Geometry: final body of the model. Coordinates: model frame, mm. Round coordinates to 2 decimals unless told otherwise and drop trailing zeros. Loops run counter-clockwise (first coordinate to the right, second up) from the corner with the lowest first, then second, coordinate; pieces in that order, holes last. Notation, with made-up numbers: (65.5, -9) -> (85.5, -9) arc R22 cw to (85.5, 12) -> close; hole circle Ø3 at (-29.75, 30.5). An arc over 180 degrees is marked (long way). Answer in a Markdown table with one row per item.
```python
from build123d import *

# Parameters (mm, degrees)
SKETCH1_W           = 67.3
SKETCH1_H           = 135.4
BOSS_EXTRUDE1_DEPTH = 15.1
FILLET1_R           = 5
FILLET2_R           = 3.75
SKETCH2_W           = 12.2
SKETCH2_H           = 4.45
CUT_EXTRUDE1_DEPTH  = 3
SKETCH3_W           = 8.2
SKETCH3_H           = 3.5
SKETCH3_W_2         = 8
SKETCH3_H_2         = 3.3
CUT_EXTRUDE2_DEPTH  = 3
FILLET3_R           = 3.75
SKETCH4_W           = 8
SKETCH4_H           = 3.3
BOSS_EXTRUDE2_DEPTH = 0.5
FILLET4_R           = 0.2
FILLET5_R           = 0.2


with BuildPart() as part:
    # Sketch1 → Boss-Extrude1 (new body)
    with BuildSketch(Plane(origin=(0, 0, 0), x_dir=(1, 0, 0), z_dir=(0, 1, 0))):
        with Locations((33.65, 67.7)):
            Rectangle(SKETCH1_W, SKETCH1_H)
    extrude(amount=BOSS_EXTRUDE1_DEPTH)

    # Fillet1
    fillet1_edges = [part.edges().sort_by_distance(p)[0] for p in [
        (0, 7.55, -135.4),
        (67.3, 7.55, -135.4),
        (67.3, 7.55, 0),
        (0, 7.55, 0),
    ]]
    fillet(fillet1_edges, radius=FILLET1_R)

    # Fillet2
    fillet2_edges = [part.edges().sort_by_distance(p)[0] for p in [
        (0, 15.1, -67.7),
        (33.65, 15.1, -135.4),
        (33.65, 15.1, 0),
        (67.3, 15.1, -67.7),
        (1.464466094, 15.1, -1.464466094),
        (65.835533906, 15.1, -1.464466094),
        (65.835533906, 15.1, -133.935533906),
        (1.464466094, 15.1, -133.935533906),
    ]]
    fillet(fillet2_edges, radius=FILLET2_R)

    # Sketch2 → Cut-Extrude1 (cut)
    with BuildSketch(Plane.XY):
        with Locations((17.1, 8.125)):
            Rectangle(SKETCH2_W, SKETCH2_H)
        with Locations((50.2, 8.125)):
            Rectangle(SKETCH2_W, SKETCH2_H)
        with BuildLine():
            Line((30.2, 7.55), (37.1, 7.55))
            ThreePointArc((37.1, 7.55), (37.807106781, 7.842893219), (38.1, 8.55))
            Line((38.1, 8.55), (38.1, 9.35))
            ThreePointArc((38.1, 9.35), (37.807106781, 10.057106781), (37.1, 10.35))
            Line((37.1, 10.35), (30.2, 10.35))
            ThreePointArc((30.2, 10.35), (29.492893219, 10.057106781), (29.2, 9.35))
            Line((29.2, 9.35), (29.2, 8.55))
            ThreePointArc((29.2, 8.55), (29.492893219, 7.842893219), (30.2, 7.55))
        make_face()
    extrude(amount=-CUT_EXTRUDE1_DEPTH, mode=Mode.SUBTRACT)

    # Sketch3 → Cut-Extrude2 (cut)
    with BuildSketch(Plane(origin=(67.3, 0, 0), x_dir=(0, 0, -1), z_dir=(1, 0, 0))):
        with Locations((15.6, 7.6)):
            Rectangle(SKETCH3_W, SKETCH3_H)
        with Locations((15.6, 7.6)):
            Rectangle(SKETCH3_W_2, SKETCH3_H_2, mode=Mode.SUBTRACT)
    extrude(amount=-CUT_EXTRUDE2_DEPTH, mode=Mode.SUBTRACT)

    # Fillet3
    fillet3_edges = [part.edges().sort_by_distance(p)[0] for p in [
        (0, 0, -67.7),
        (33.65, 0, -135.4),
        (67.3, 0, -67.7),
        (33.65, 0, 0),
        (1.464466094, 0, -1.464466094),
        (65.835533906, 0, -1.464466094),
        (65.835533906, 0, -133.935533906),
        (1.464466094, 0, -133.935533906),
    ]]
    fillet(fillet3_edges, radius=FILLET3_R)

    # Sketch4 → Boss-Extrude2 (add)
    with BuildSketch(Plane(origin=(67.3, 0, 0), x_dir=(0, 0, -1), z_dir=(1, 0, 0))):
        with Locations((15.6, 7.6)):
            Rectangle(SKETCH4_W, SKETCH4_H)
    extrude(amount=BOSS_EXTRUDE2_DEPTH)

    # Fillet4
    fillet4_edges = [part.edges().sort_by_distance(p)[0] for p in [
        (66.05, 9.25, -11.6),
        (66.05, 9.25, -19.6),
        (66.05, 5.95, -19.6),
        (66.05, 5.95, -11.6),
    ]]
    fillet(fillet4_edges, radius=FILLET4_R)

    # Fillet5
    fillet5_edges = [part.edges().sort_by_distance(p)[0] for p in [
        (67.8, 7.6, -11.6),
        (67.8, 5.95, -15.6),
        (67.8, 7.6, -19.6),
        (67.8, 9.25, -15.6),
        (67.8, 9.191421356, -11.658578644),
        (67.8, 9.191421356, -19.541421356),
        (67.8, 6.008578644, -19.541421356),
        (67.8, 6.008578644, -11.658578644),
    ]]
    fillet(fillet5_edges, radius=FILLET5_R)


solid = part.part
```
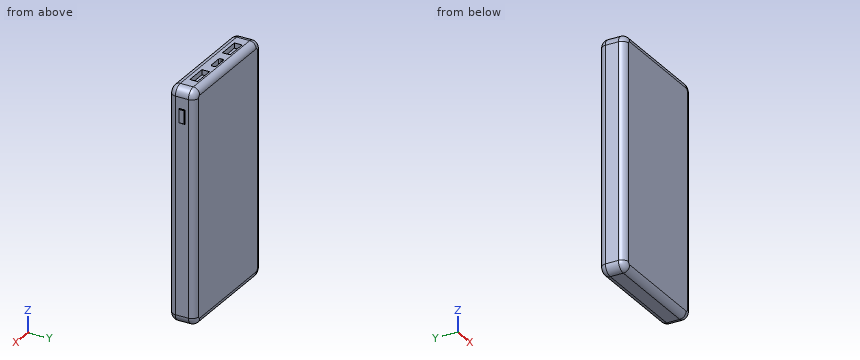
Item 1: Section query A-A, the plane z = -55. Output: boundary loops of the cut face in (x, y), and give its area (3 significant figures).
Ans:
| item | result |
|---|---|
| outline | (0, 3.75) arc R3.75 ccw to (3.75, 0) -> (63.55, 0) arc R3.75 ccw to (67.3, 3.75) -> (67.3, 11.35) arc R3.75 ccw to (63.55, 15.1) -> (3.75, 15.1) arc R3.75 ccw to (0, 11.35) -> close |
| area | 1,000 mm2 |
Item 2: First-contact query: P1, Ø3.5, axis at x = 66, z = -15.5, coming from the -Y side; P2, Ø3, axis at x = 65.5, y = 8, coming from the +Z side; P3, Ø3.5, axis at x = 35, z = -1.5, coming from the -Y side. Flat tips, straight axial feed; report the tip coordinate or a pass-through.
Ans:
| item | result |
|---|---|
| P1 | y = 0.07 |
| P2 | z = -0.3 |
| P3 | y = 0.03 |
Item 3: Ray query, L1, parallel to Z at x = 37.5, y = 8; L2, parallel to Z at x = 43, y = 11.5; L3, parallel to X at y = 4.25, z = -102.5. Return the intervals inside material, ascending.
Ans:
| item | result |
|---|---|
| L1 | -135.4 to -3 |
| L2 | -135.4 to 0 |
| L3 | 0 to 67.3 |
